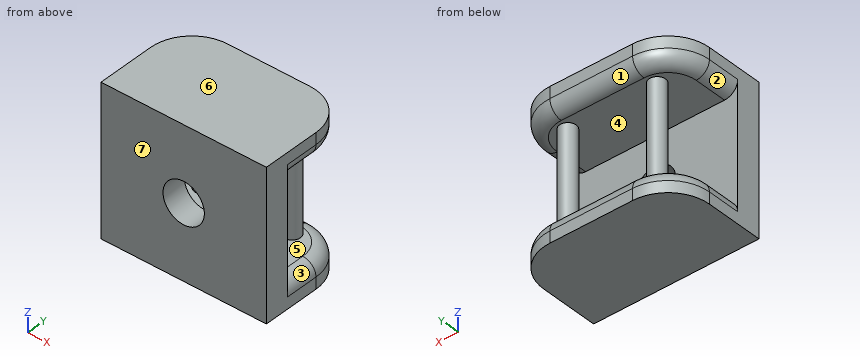
```python
from build123d import *

# Parameters (mm, degrees)
BOSS_EXTRUDE1_DEPTH = 100
SKETCH2_R           = 5
BOSS_EXTRUDE2_DEPTH = 60
SKETCH3_R           = 12.5
CUT_EXTRUDE1_DEPTH  = 148.309198627
CUT_EXTRUDE2_DEPTH  = 148.309198627
FILLET1_R           = 8


with BuildPart() as part:
    # Sketch1 → Boss-Extrude1 (new body)
    with BuildSketch(Plane(origin=(0, 0, 0), x_dir=(0, 0, -1), z_dir=(1, 0, 0))):
        Polygon((0, 0), (0, 60), (15, 60), (15, 15), (75, 15), (75, 60), (90, 60), (90, 0), align=None)
    extrude(amount=BOSS_EXTRUDE1_DEPTH)

    # Sketch2 → Boss-Extrude2 (add)
    with BuildSketch(Plane(origin=(0, 0, -15), x_dir=(-1, 0, 0), z_dir=(0, 0, -1))):
        with Locations(Location((-77, 45, 0), (0, 0, 270))):
            Circle(SKETCH2_R)
        with Locations(Location((-23, 45, 0), (0, 0, 270))):
            Circle(SKETCH2_R)
    extrude(amount=BOSS_EXTRUDE2_DEPTH)

    # Sketch3 → Cut-Extrude1 (cut, through all)
    with BuildSketch(Plane.XZ):
        with Locations(Location((50, -45, 0), (0, 0, 270))):
            Circle(SKETCH3_R)
    extrude(amount=-CUT_EXTRUDE1_DEPTH, mode=Mode.SUBTRACT)

    # Sketch4 → Cut-Extrude2 (cut, through all)
    with BuildSketch(Plane(origin=(0, 0, -90), x_dir=(-1, 0, 0), z_dir=(0, 0, -1))):
        with BuildLine():
            ThreePointArc((-100, 35), (-92.67766953, 52.67766953), (-75, 60))
            Line((-75, 60), (-100, 60))
            Line((-100, 60), (-100, 35))
        make_face()
        with BuildLine():
            ThreePointArc((-25, 60), (-7.32233047, 52.67766953), (0, 35))
            Line((0, 35), (0, 60))
            Line((0, 60), (-25, 60))
        make_face()
    extrude(amount=-CUT_EXTRUDE2_DEPTH, mode=Mode.SUBTRACT)

    # Fillet1
    fillet1_edges = [part.edges().sort_by_distance(p)[0] for p in [
        (100, 25, -15),
        (0, 25, -75),
        (100, 25, -75),
        (50, 60, -15),
        (50, 60, -75),
        (92.67766953, 52.67766953, -75),
        (92.67766953, 52.67766953, -15),
        (7.32233047, 52.67766953, -75),
        (7.32233047, 52.67766953, -15),
        (0, 25, -15),
    ]]
    fillet(fillet1_edges, radius=FILLET1_R)


solid = part.part
```
Geometry check sheet. Reference: the model listing, model coordinates, mm. Face numbers are marked on the shaded views. A direction names the side the tool comes from. Coordinates: 2 decimals unless noted, no trailing zeros. Write each loop counter-clockwise with the first axis right and the second up, starting at its lowest first coordinate (ties: lowest second). Pieces come first, ordered by that corner, then holes. Notation, with made-up numbers: M -12,81.5 L -5,81.5 A19 ccw -5,90.5 Z; hole C -22.75,17.25 d3. An arc over 180 degrees is marked long. One line per item, written item: value. Start each with the question number.
(1) Sectioned sample at A-A, the plane x = 50. Enter the section's corners in (y, z).
(2) Sectioned sample at D-D, the plane z = -45. Enter the section's corners in (x, y), and give its area (3 significant figures).
(3) Release check for a two-part mould opening along Z. For the marked faces 5, 6 and 7 record: released by +Z, released by -Z, zero draft, split by the parting line, or undercut.
(4) Sectioned sample at C-C, the plane z = -24.5. Enter the section's corners in (x, y).
(5) Depth check by flat-ended pin: pin 1 (8 mm diameter, centred on y = 45.5, z = -63, fed in from +X); pin 2 (10 mm diameter, centred on y = 36, z = -38, fed in from -X); pin 3 (23 mm diameter, centred on x = 64, z = -28, fed in from +Y). Enter the tip coordinate at first touch or a pass-through.
(6) Sectioned sample at B-B, the plane y = 20. Enter the section's corners in (x, z).
(7) Scan lines: line 1 along Z through (x, y) = (32, 48); line 2 along X through (y, z) = (7, -45); line 3 along Y through (x, z) = (92, -25). Record each from-to range of solid material in increasing order. Write a range as [from, to].
(8) Tool access check on the marked faces 1, 2, 3 and 4. Record the directions out of +Z, -Z, +X, -X, +Y, -Y that give a thin tool (end or side, any length) a straight path to the whole face; none if there is none.
Filled sheet:
1. outline: M 0,-90 L 60,-90 L 60,-83 A8 ccw 52,-75 L 15,-75 L 15,-57.5 L 0,-57.5 Z; M 0,-32.5 L 15,-32.5 L 15,-15 L 52,-15 A8 ccw 60,-7 L 60,0 L 0,0 Z
2. outline: M 0,0 L 37.5,0 L 37.5,15 L 0,15 Z; C 23,45 d10; M 62.5,0 L 100,0 L 100,15 L 62.5,15 Z; C 77,45 d10
2. area: 1,280 mm²
3. face 5: undercut
3. face 6: released by +Z
3. face 7: zero draft
4. outline: M 0,0 L 100,0 L 100,15 L 0,15 Z; C 23,45 d10; C 77,45 d10
5. pin 1: x = 82
5. pin 2: x = 20
5. pin 3: y = 49.77
6. outline: M 0,-90 L 100,-90 L 100,-83 A8 ccw 92,-75 L 8,-75 A8 ccw 0,-83 Z; M 0,-7 A8 ccw 8,-15 L 92,-15 A8 ccw 100,-7 L 100,0 L 0,0 Z
7. line 1: [-90, -75], [-15, 0]
7. line 2: [0, 37.5], [62.5, 100]
7. line 3: [0, 15]
8. face 1: +X, -X, +Y
8. face 2: -X, +Y
8. face 3: +X, +Y
8. face 4: none
